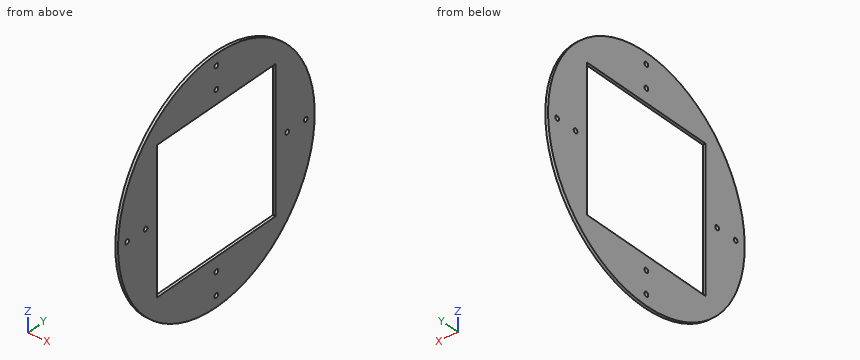
from build123d import *

# Parameters (mm, degrees)
SKETCH1_R           = 86.487
BOSS_EXTRUDE1_DEPTH = 2.0066
SKETCH6_W           = 104.14
SKETCH6_H           = 104.14
CUT_EXTRUDE2_DEPTH  = 123.327547108
SKETCH7_R           = 1.651
CUT_EXTRUDE3_DEPTH  = 123.327547108
CIRPATTERN1_COUNT   = 4


with BuildPart() as part:
    # Sketch1 → Boss-Extrude1 (new body)
    with BuildSketch(Plane.YZ):
        with Locations(Location((0, 0, 0), (0, 0, 270))):
            Circle(SKETCH1_R)
    extrude(amount=BOSS_EXTRUDE1_DEPTH)

    # Sketch6 → Cut-Extrude2 (cut, through all)
    with BuildSketch(Plane(origin=(2.0066, 0, 0), x_dir=(0, 0, -1), z_dir=(1, 0, 0))):
        Rectangle(SKETCH6_W, SKETCH6_H)
    extrude(amount=-CUT_EXTRUDE2_DEPTH, mode=Mode.SUBTRACT)

    # Sketch7 → Cut-Extrude3 (cut, through all)
    with BuildSketch(Plane.YZ.offset(2.0066)):
        with Locations(Location((62.23, 0, 0), (0, 0, 270))):
            Circle(SKETCH7_R)
        with Locations(Location((78.486, 0, 0), (0, 0, 270))):
            Circle(SKETCH7_R)
    cut_extrude3 = extrude(amount=-CUT_EXTRUDE3_DEPTH, mode=Mode.SUBTRACT)

    # CirPattern1: Cut-Extrude3 ×4 about axis
    cirpattern1_axis = Axis((0, 0, 0), (1, 0, 0))
    for i in range(1, CIRPATTERN1_COUNT):
        add(cut_extrude3.rotate(cirpattern1_axis, i * 360 / CIRPATTERN1_COUNT), mode=Mode.SUBTRACT)


solid = part.part
Geometry check sheet. Reference: the model listing, model coordinates, mm. Give positions to 0.01 mm unless a question says otherwise; leave off trailing zeros. Order: outer loops, then holes, each group sorted by start corner. A loop starts at its lowest first (then second) coordinate and runs counter-clockwise, first axis right, second up.
1) Material ranges on probe 1 along Y at (x, z) = (0.9, 0) (3 decimals); probe 2 along Z at (x, y) = (0.5, -62.23); probe 3 along Z at (x, y) = (0.1, 30.5), recorded low to high.
Results are:
probe 1: y = -86.487 to -80.137, -76.835 to -63.881, -60.579 to -52.07, 52.07 to 60.579, 63.881 to 76.835, 80.137 to 86.487
probe 2: z = -60.06 to -1.65, 1.65 to 60.06
probe 3: z = -80.93 to -52.07, 52.07 to 80.93
2) Cross-section at B-B (z = -44). Record the boundary of the cut face in (x, y).
Results are:
outline: (0, -74.46) - (2.01, -74.46) - (2.01, -52.07) - (0, -52.07) - close; (0, 52.07) - (2.01, 52.07) - (2.01, 74.46) - (0, 74.46) - close
3) Cross-section at A-A (x = 1.15). Give the number of separate pieces and of enclosed holes in the cut face, then the cut area to 3 significant figures.
Results are:
separate pieces: 1
enclosed holes: 9
area: 12,600 mm2
4) Gauge pin test, flat ends, axial feed: pin 1 (6 mm diameter, centred on y = 48.5, z = -42, fed in from +X); pin 2 (1 mm diameter, centred on x = 0.5, y = 19, fed in from +Z); pin 3 (0.6 mm diameter, centred on x = 1.5, y = -3, fed in from -Z). Record the tip position at first contact, or that the pin passes through.
Results are:
pin 1: passes through
pin 2: stops at z = 84.49
pin 3: stops at z = -86.44
5) Cross-section at D-D (z = -68). Record the boundary of the cut face in (x, y), then the cut area to 3 significant figures.
Results are:
outline: (0, -53.44) - (2.01, -53.44) - (2.01, 53.44) - (0, 53.44) - close
area: 214 mm2
6) Cross-section at C-C (y = 40). Record the boundary of the cut face in (x, z).
Results are:
outline: (0, -76.68) - (2.01, -76.68) - (2.01, -52.07) - (0, -52.07) - close; (0, 52.07) - (2.01, 52.07) - (2.01, 76.68) - (0, 76.68) - close
